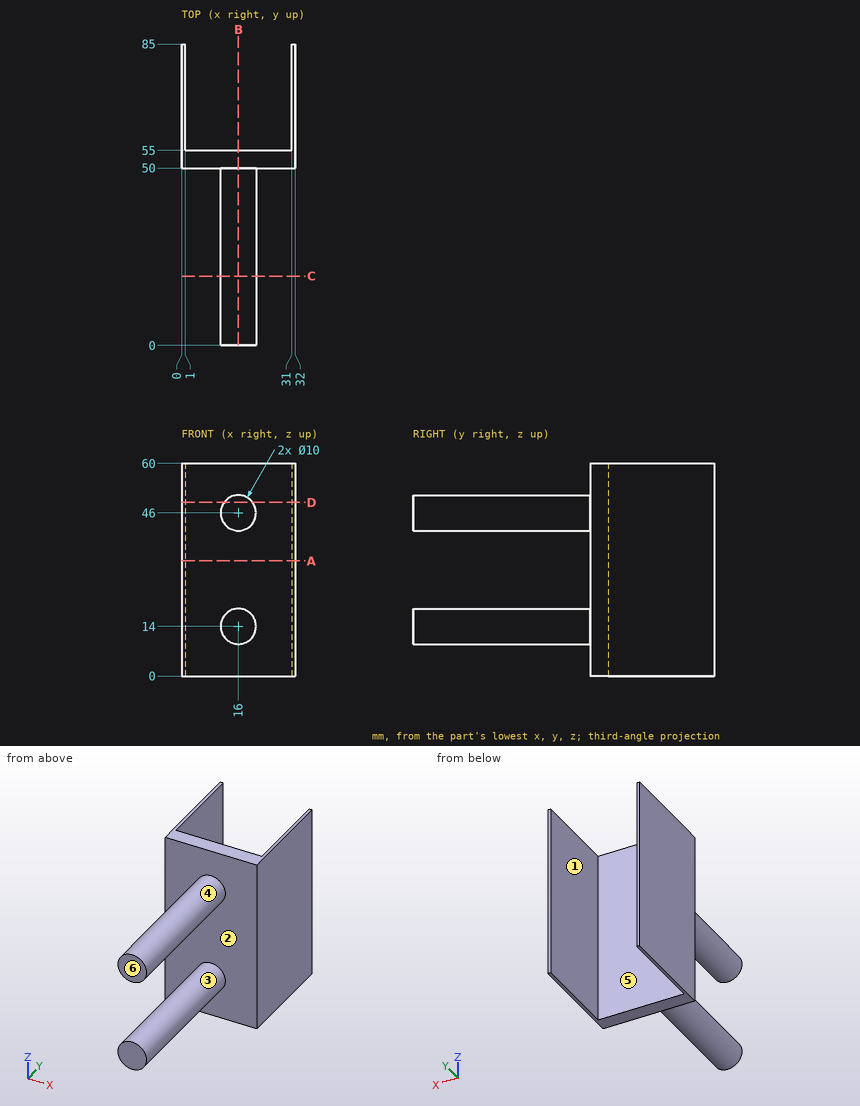
Input: dimensioned drawing with shaded views. Units: mm. Origin: part minimum x, y, z. A direction names the side the tool comes from. Coordinates: 2 decimals unless noted, no trailing zeros. Loops run counter-clockwise (first coordinate to the right, second up) from the corner with the lowest first, then second, coordinate; pieces in that order, holes last. Notation, with made-up numbers: M 86.5,-34.75 L 124.5,-34.75 A17 ccw 124.5,-17.75 Z; hole C 12.25,61 d3. An arc over 180 degrees is marked long. Use a Markdown table: item, result. Add a question column.
1) Section C-C, the plane y = 19.5. Return the cut outline in (x, z).
2) Section A-A, the plane z = 32.5. Return the cut outline in (x, y), plus the area to 3 significant figures.
3) Pin query (flat end, axial travel): P1, Ø9, axis at x = 11, z = 18.5, coming from the +Y side; P2, Ø10, axis at x = 6.5, y = 62, coming from the +Z side; P3, Ø12, axis at x = 6.5, z = 38.5, coming from the -Y side; P4, Ø1, axis at x = 11, y = 24.5, coming from the -Z side. Return the tip coordinate at first contact, or that it passes through.
4) Draft query along Z for the marked faces 1, 2 and 3. Return one class per face: +Z half, -Z half, draft (parallel to the pull), parting line (faces both ways), or undercut.
5) Section D-D, the plane z = 49. Return the cut outline in (x, y).
6) Set-up query: the marked faces 4, 5 and 6. Return all of +Z, -Z, +X, -X, +Y, -Y with unobstructed straight access to the full face (end or side cutting, diameter ignored); none if empty.
7) Line query: L1, parallel to X at y = 80.5, z = 18; L2, parallel to Y at x = 16.5, z = 34.5; L3, parallel to Y at x = 17, z = 43. Output: solid intervals per line, ascending. Write a range as from..to.
8) Section B-B, the plane x = 16. Return the cut outline in (y, z).
Answer below:
| question | item | result |
|---|---|---|
| 1 | outline | C 16,14 d10; C 16,46 d10 |
| 2 | outline | M 0,50 L 32,50 L 32,85 L 31,85 L 31,55 L 1,55 L 1,85 L 0,85 Z |
| 2 | area | 220 mm2 |
| 3 | P1 | y = 55 |
| 3 | P2 | through |
| 3 | P3 | y = 50 |
| 3 | P4 | z = 11.82 |
| 4 | face 1 | draft |
| 4 | face 2 | undercut |
| 4 | face 3 | undercut |
| 5 | outline | M 0,50 L 12,50 L 12,0 L 20,0 L 20,50 L 32,50 L 32,85 L 31,85 L 31,55 L 1,55 L 1,85 L 0,85 Z |
| 6 | face 4 | -Y |
| 6 | face 5 | +Z, -Z, +Y |
| 6 | face 6 | +Z, -Z, +X, -X, -Y |
| 7 | L1 | 0..1, 31..32 |
| 7 | L2 | 50..55 |
| 7 | L3 | 0..55 |
| 8 | outline | M 0,9 L 50,9 L 50,0 L 55,0 L 55,60 L 50,60 L 50,51 L 0,51 L 0,41 L 50,41 L 50,19 L 0,19 Z |
